Input: part model. Units: mm. Frame: model coordinates. Face numbers are marked on the shaded views. Coordinates: 2 decimals unless noted, no trailing zeros. Write each loop counter-clockwise with the first axis right and the second up, starting at its lowest first coordinate (ties: lowest second). Pieces come first, ordered by that corner, then holes. Notation, with made-up numbers: M 34,-30.5 L 60,-30.5 A17 ccw 60,-6.5 Z; hole C 73.5,88 d3. An arc over 180 degrees is marked long. Answer as a JSON object with one key per item and string values. Group by question number.
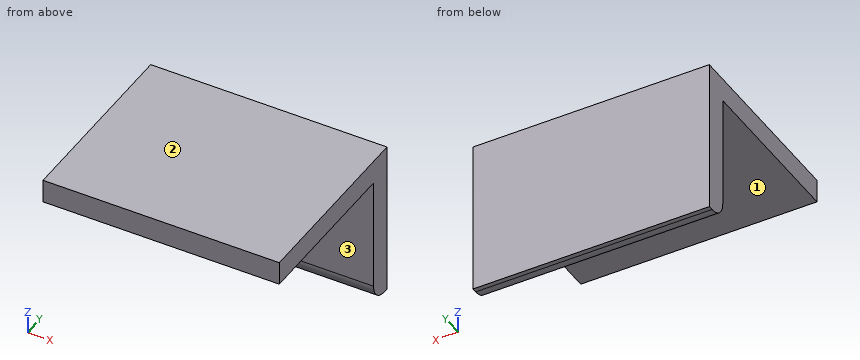
from build123d import *

# Parameters (mm, degrees)
SKETCH1_W           = 50
SKETCH1_H           = 40
BOSS_EXTRUDE1_DEPTH = 5
SKETCH2_W           = 50
SKETCH2_H           = 5
BOSS_EXTRUDE2_DEPTH = 28
FILLET1_R           = 4


with BuildPart() as part:
    # Sketch1 → Boss-Extrude1 (new body)
    with BuildSketch(Plane.XY):
        Rectangle(SKETCH1_W, SKETCH1_H)
    extrude(amount=BOSS_EXTRUDE1_DEPTH)

    # Sketch2 → Boss-Extrude2 (add)
    with BuildSketch(Plane(origin=(0, 0, 0), x_dir=(-1, 0, 0), z_dir=(0, 0, -1))):
        with Locations((0, 17.5)):
            Rectangle(SKETCH2_W, SKETCH2_H)
    extrude(amount=BOSS_EXTRUDE2_DEPTH)

    # Fillet1
    fillet1_edges = [part.edges().sort_by_distance(p)[0] for p in [
        (0, 15, -28),
    ]]
    fillet(fillet1_edges, radius=FILLET1_R)


solid = part.part
Q1. Section B-B, the plane z = -23. Return the cut outline in (x, y).
Q2. Pin query (flat end, axial travel): pin 1 Ø10 at (y, z) = (2, -8.5) entering from -X; pin 2 Ø17.5 at (x, y) = (6.5, 0.5) entering from -Z; pin 3 Ø12 at (x, z) = (8, -12) entering from -Y. Return the tip coordinate at first contact, or that it passes through.
Q3. Section A-A, the plane x = -8. Return the cut outline in (y, z), and give its area (3 significant figures).
Q4. Section C-C, the plane y = -17. Return the cut outline in (x, z).
Q5. Line query: line 1 (Y direction, x = 14.5, z = -11); line 2 (Z direction, x = 7, y = 5.5); line 3 (Y direction, x = -8, z = -25). Output: solid intervals per line, ascending. Write a range as from..to.
Q6. Draft query along Z for the marked faces 1, 2 and 3. Return one class per face: released by +Z, released by -Z, zero draft, split by the parting line, or undercut.
Filled in:
{
 "1": {"outline": "M -25,15 L 25,15 L 25,20 L -25,20 Z"},
 "2": {"pin 1": "through", "pin 2": "z = 0", "pin 3": "y = 15"},
 "3": {"outline": "M -20,0 L 15,0 L 15,-24 A4 ccw 19,-28 L 20,-28 L 20,5 L -20,5 Z", "area": "337 mm^2"},
 "4": {"outline": "M -25,0 L 25,0 L 25,5 L -25,5 Z"},
 "5": {"line 1": "15..20", "line 2": "0..5", "line 3": "15.13..20"},
 "6": {"face 1": "released by -Z", "face 2": "released by +Z", "face 3": "zero draft"}
}
